For this review, use the dimensioned drawing (mm, ordinates from the lowest corner) and the shaded views. Round coordinates to 2 decimals unless told otherwise and drop trailing zeros. Order: outer loops, then holes, each group sorted by start corner. A loop starts at its lowest first (then second) coordinate and runs counter-clockwise, first axis right, second up. Notation, with made-up numbers: (31, 48.25) -> (56, 48.25) arc R14 ccw to (56, 69.25) -> close; hole circle Ø11 at (-17.5, -40). An arc over 180 degrees is marked (long way). Answer in a Markdown table with one row per item.
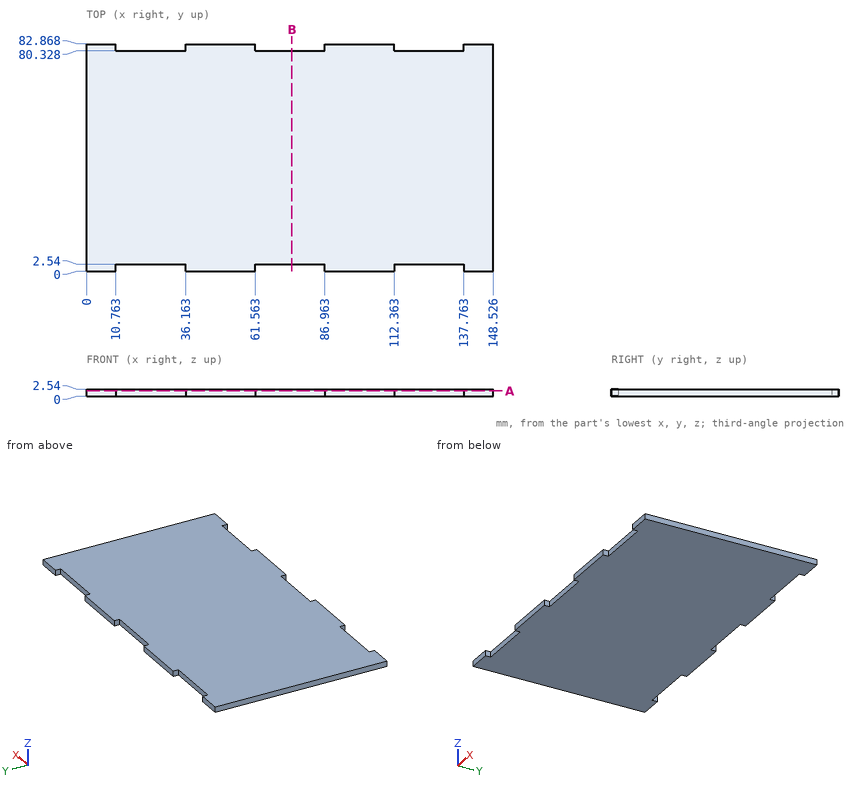
Q1. To check wall thickness, follow probe 1 along Y at (x, z) = (85, 1.95). State the ranges of the line that lie inside material, in increasing order.
Answer key:
| item | result |
|---|---|
| probe 1 | y = 2.54 to 80.33 |
Q2. Take a section at A-A, the plane z = 1.9. Write out the cut boundary in (x, y).
Answer key:
| item | result |
|---|---|
| outline | (0, 0) -> (10.76, 0) -> (10.76, 2.54) -> (36.16, 2.54) -> (36.16, 0) -> (61.56, 0) -> (61.56, 2.54) -> (86.96, 2.54) -> (86.96, 0) -> (112.36, 0) -> (112.36, 2.54) -> (137.76, 2.54) -> (137.76, 0) -> (148.53, 0) -> (148.53, 82.87) -> (137.76, 82.87) -> (137.76, 80.33) -> (112.36, 80.33) -> (112.36, 82.87) -> (86.96, 82.87) -> (86.96, 80.33) -> (61.56, 80.33) -> (61.56, 82.87) -> (36.16, 82.87) -> (36.16, 80.33) -> (10.76, 80.33) -> (10.76, 82.87) -> (0, 82.87) -> close |
Q3. Clearance check with flat-ended pins moving along their axes: pin 1 Ø1.3 at (x, z) = (127, 1) entering from +Y; pin 2 Ø1 at (x, z) = (84, 2) entering from -Y. State where each tip first meets the part, or that it passes through.
Answer key:
| item | result |
|---|---|
| pin 1 | stops at y = 80.33 |
| pin 2 | stops at y = 2.54 |
Q4. Take a section at B-B, the plane x = 75. Write out the cut boundary in (y, z).
Answer key:
| item | result |
|---|---|
| outline | (2.54, 0) -> (80.33, 0) -> (80.33, 2.54) -> (2.54, 2.54) -> close |
